Here's the drawing with two shaded views (mm, measured from the low corner). I have some questions. Round coordinates to 2 decimals unless told otherwise and drop trailing zeros. Loops run counter-clockwise (first coordinate to the right, second up) from the corner with the lowest first, then second, coordinate; pieces in that order, holes last. Notation, with made-up numbers: (41, 18.5) -> (50, 18.5) arc R22 ccw to (50, 33.5) -> close; hole circle Ø10 at (5, -21.75). An arc over 180 degrees is marked (long way). Use a Markdown table: item, result.
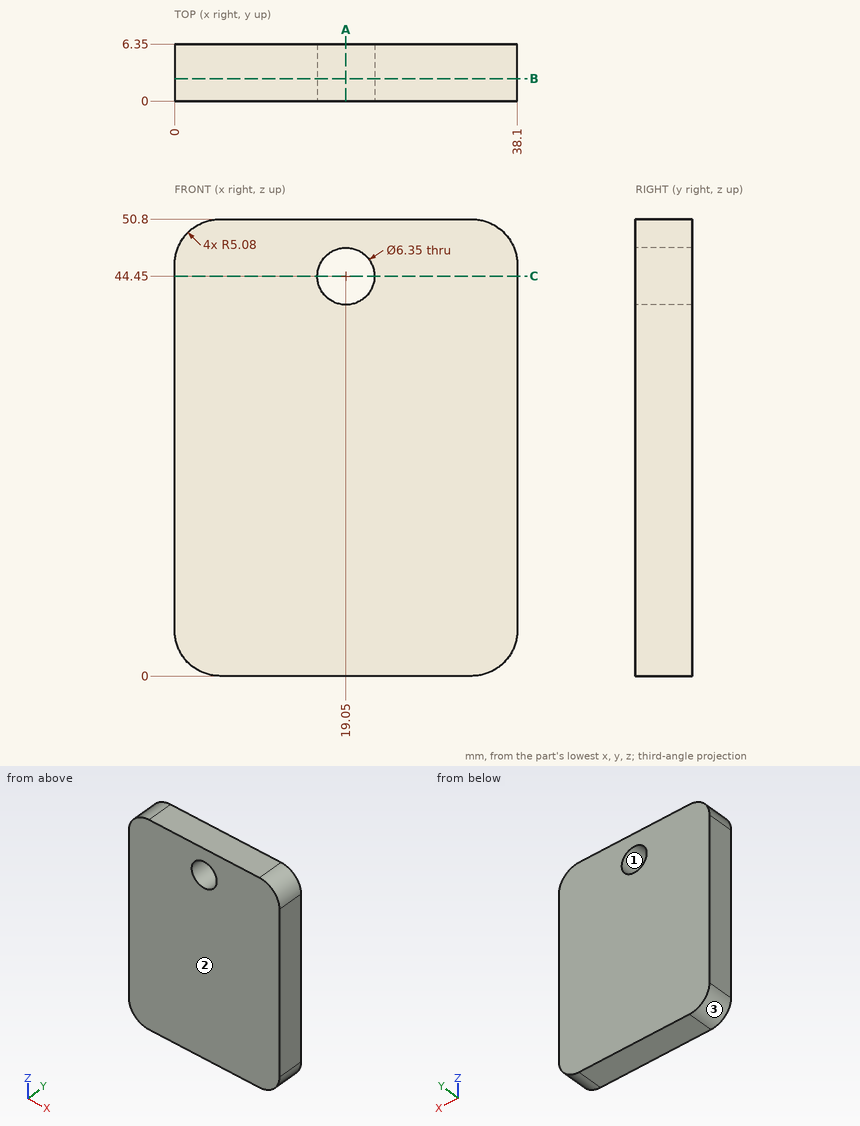
1. I need wall thicknesses on line 1 (X direction, y = 2.75, z = 44.45) (3 decimals); line 2 (X direction, y = 5.5, z = 5); line 3 (Z direction, x = 16.5, y = 1.5). Which ranges of each line are inside material? Lowest first, please.
Answer sheet:
| item | result |
|---|---|
| line 1 | x = 0 to 15.875, 22.225 to 38.1 |
| line 2 | x = 0 to 38.1 |
| line 3 | z = 0 to 42.56, 46.34 to 50.8 |
2. I want a section at C-C (z = 44.45). Please give me the cut outline in (x, y) (3 decimals).
Answer sheet:
| item | result |
|---|---|
| outline | (0, 0) -> (15.875, 0) -> (15.875, 6.35) -> (0, 6.35) -> close; (22.225, 0) -> (38.1, 0) -> (38.1, 6.35) -> (22.225, 6.35) -> close |
3. I want a section at B-B (y = 2.5). Please give me the cut outline in (x, z) (3 decimals), plus the area to 3 significant figures.
Answer sheet:
| item | result |
|---|---|
| outline | (0, 5.08) arc R5.08 ccw to (5.08, 0) -> (33.02, 0) arc R5.08 ccw to (38.1, 5.08) -> (38.1, 45.72) arc R5.08 ccw to (33.02, 50.8) -> (5.08, 50.8) arc R5.08 ccw to (0, 45.72) -> close; hole circle Ø6.35 at (19.05, 44.45) |
| area | 1,880 mm² |
4. Will this pin go through, and if not, where does the flat tip stop? pin 1 Ø5.5 at (x, z) = (19.05, 44.45) entering from +Y.
Answer sheet:
| item | result |
|---|---|
| pin 1 | passes through |
5. If we mould it in two halves opening along Z, with no side actions, what happens to the marked faces 1, 2 and 3? For each: +Z half, -Z half, draft (parallel to the pull), parting line (faces both ways), or undercut.
Answer sheet:
| item | result |
|---|---|
| face 1 | undercut |
| face 2 | draft |
| face 3 | -Z half |
6. I want a section at A-A (x = 19.05). Please give me the cut outline in (y, z) (3 decimals), plus the area to 3 significant figures.
Answer sheet:
| item | result |
|---|---|
| outline | (0, 0) -> (6.35, 0) -> (6.35, 41.275) -> (0, 41.275) -> close; (0, 47.625) -> (6.35, 47.625) -> (6.35, 50.8) -> (0, 50.8) -> close |
| area | 282 mm² |
